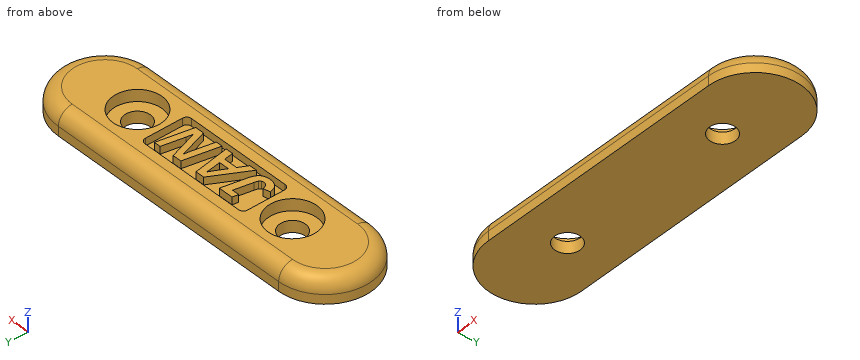
from build123d import *

# Parameters (mm, degrees)
F0_R     = 5.25
F0_R_2   = 2.75
F1_DEPTH = 5
F2_DEPTH = 2.5
F4_R     = 3
F6_DEPTH = 1.6


with BuildPart() as f1:
    # F0 (on Top) → F1 (new body)
    with BuildSketch(Plane.XY):
        with BuildLine():
            Line((27, 10), (-27, 10))
            ThreePointArc((-27, 10), (-37, 0), (-27, -10))
            Line((-27, -10), (27, -10))
            ThreePointArc((27, -10), (37, 0), (27, 10))
        make_face()
        with Locations((-19, 0)):
            Circle(F0_R, mode=Mode.SUBTRACT)
        with Locations((19, 0)):
            Circle(F0_R, mode=Mode.SUBTRACT)
        with Locations((-19, 0)):
            Circle(F0_R)
        with Locations((-19, 0)):
            Circle(F0_R_2, mode=Mode.SUBTRACT)
        with Locations((19, 0)):
            Circle(F0_R)
        with Locations((19, 0)):
            Circle(F0_R_2, mode=Mode.SUBTRACT)
    extrude(amount=-F1_DEPTH)

    # F0 (on Top) → F2 (cut)
    with BuildSketch(Plane.XY):
        with Locations((-19, 0)):
            Circle(F0_R)
        with Locations((-19, 0)):
            Circle(F0_R_2, mode=Mode.SUBTRACT)
        with Locations((19, 0)):
            Circle(F0_R)
        with Locations((19, 0)):
            Circle(F0_R_2, mode=Mode.SUBTRACT)
    extrude(amount=-F2_DEPTH, mode=Mode.SUBTRACT)

    # F4
    f4_edges = [f1.edges().sort_by_distance(p)[0] for p in [
        (0, -10, 0),
        (0, 10, 0),
    ]]
    fillet(f4_edges, radius=F4_R)

    # F5 (on face) → F6 (cut)
    with BuildSketch(Plane.XY):
        with BuildLine():
            Line((11.5, 5), (-11.5, 5))
            ThreePointArc((-11.5, 5), (-12.2071067812, 4.7071067812), (-12.5, 4))
            Line((-12.5, 4), (-12.5, -4))
            ThreePointArc((-12.5, -4), (-12.2071067812, -4.7071067812), (-11.5, -5))
            Line((-11.5, -5), (11.5, -5))
            ThreePointArc((11.5, -5), (12.2071067812, -4.7071067812), (12.5, -4))
            Line((12.5, -4), (12.5, 4))
            ThreePointArc((12.5, 4), (12.2071067812, 4.7071067812), (11.5, 5))
        make_face()
        with BuildLine():
            add(Edge.make_bspline(
                [(-7.1087151842, -3.5052785265), (-7.754492363, -4.0761455526), (-8.9168912848, -4.0761455526)],
                knots=[0, 0, 0, 1, 1, 1], degree=2))
            add(Edge.make_bspline(
                [(-8.9168912848, -4.0761455526), (-9.939802336, -4.0761455526), (-10.5502770291, -3.5586627733)],
                knots=[0, 0, 0, 1, 1, 1], degree=2))
            add(Edge.make_bspline(
                [(-10.5502770291, -3.5586627733), (-11.1607517221, -3.041179994), (-11.3656783468, -1.928721174)],
                knots=[0, 0, 0, 1, 1, 1], degree=2))
            Line((-11.3656783468, -1.928721174), (-9.9277478287, -1.6153039832))
            add(Edge.make_bspline(
                [(-9.9277478287, -1.6153039832), (-9.6814914645, -2.8328092243), (-8.8152890087, -2.8328092243)],
                knots=[0, 0, 0, 1, 1, 1], degree=2))
            add(Edge.make_bspline(
                [(-8.8152890087, -2.8328092243), (-8.5242587601, -2.8328092243), (-8.325359389, -2.7036537886)],
                knots=[0, 0, 0, 1, 1, 1], degree=2))
            add(Edge.make_bspline(
                [(-8.325359389, -2.7036537886), (-8.126460018, -2.5744983528), (-7.9973045822, -2.3377133872)],
                knots=[0, 0, 0, 1, 1, 1], degree=2))
            add(Edge.make_bspline(
                [(-7.9973045822, -2.3377133872), (-7.8681491465, -2.1009284217), (-7.7699910153, -1.5998053309)],
                knots=[0, 0, 0, 1, 1, 1], degree=2))
            Line((-7.7699910153, -1.5998053309), (-7.0002246181, 2.3712938005))
            Line((-7.0002246181, 2.3712938005), (-8.5139263252, 2.3712938005))
            Line((-8.5139263252, 2.3712938005), (-8.2762803235, 3.6146301288))
            Line((-8.2762803235, 3.6146301288), (-5.1817160827, 3.6146301288))
            Line((-5.1817160827, 3.6146301288), (-6.2201257862, -1.6910751722))
            add(Edge.make_bspline(
                [(-6.2201257862, -1.6910751722), (-6.4629380054, -2.9344115004), (-7.1087151842, -3.5052785265)],
                knots=[0, 0, 0, 1, 1, 1], degree=2))
        make_face(mode=Mode.SUBTRACT)
        Polygon((1.7909553759, -3.9676549865), (0.220425277, -3.9676549865), (-0.075771189, -2.0303234501), (-2.965408805, -2.0303234501), (-4.0141509434, -3.9676549865), (-5.5967355496, -3.9676549865), (-1.3621593291, 3.6146301288), (0.5114555256, 3.6146301288), align=None, mode=Mode.SUBTRACT)
        with BuildLine():
            Line((9.2613057802, -3.9676549865), (7.346361186, -3.9676549865))
            Line((7.346361186, -3.9676549865), (5.3332584606, 2.1181491465))
            add(Edge.make_bspline(
                [(5.3332584606, 2.1181491465), (5.2092692423, 1.2467804732), (5.1283318359, 0.8334830788)],
                knots=[0, 0, 0, 1, 1, 1], degree=2))
            Line((5.1283318359, 0.8334830788), (4.1915244085, -3.9676549865))
            Line((4.1915244085, -3.9676549865), (2.7828691225, -3.9676549865))
            Line((2.7828691225, -3.9676549865), (4.2569631626, 3.6146301288))
            Line((4.2569631626, 3.6146301288), (6.1409104522, 3.6146301288))
            Line((6.1409104522, 3.6146301288), (8.1695118299, -2.524558251))
            Line((8.1695118299, -2.524558251), (8.2332285115, -2.0837076969))
            add(Edge.make_bspline(
                [(8.2332285115, -2.0837076969), (8.2935010482, -1.6376909254), (8.3899371069, -1.1469002695)],
                knots=[0, 0, 0, 1, 1, 1], degree=2))
            Line((8.3899371069, -1.1469002695), (9.3267445343, 3.6146301288))
            Line((9.3267445343, 3.6146301288), (10.7353998203, 3.6146301288))
            Line((10.7353998203, 3.6146301288), (9.2613057802, -3.9676549865))
        make_face(mode=Mode.SUBTRACT)
        with BuildLine():
            add(Edge.make_bspline(
                [(-0.559673555, 1.596361186), (-0.6561096137, 2.3230757712), (-0.6561096137, 2.4470649895)],
                knots=[0, 0, 0, 1, 1, 1], degree=2))
            add(Edge.make_bspline(
                [(-0.6561096137, 2.4470649895), (-0.7697663971, 2.1026504942), (-1.184785864, 1.3070530099)],
                knots=[0, 0, 0, 1, 1, 1], degree=2))
            Line((-1.184785864, 1.3070530099), (-2.3247978437, -0.8352051512))
            Line((-2.3247978437, -0.8352051512), (-0.1997604073, -0.8352051512))
            Line((-0.1997604073, -0.8352051512), (-0.559673555, 1.596361186))
        make_face()
    extrude(amount=-F6_DEPTH, mode=Mode.SUBTRACT)


solid = f1.part
Source: CAD feature listing. Evaluate the final solid. Frame: model axes, mm. Give positions to 0.01 mm unless a question says otherwise; leave off trailing zeros. Write each loop counter-clockwise with the first axis right and the second up, starting at its lowest first coordinate (ties: lowest second). Pieces come first, ordered by that corner, then holes. Notation, with made-up numbers: M 9,18 L 44,18 A38 cw 44,56 Z; hole C 55.5,85 d6. An arc over 180 degrees is marked long. Return JSON: item names as keys, results as strings. Group by question number.
1) Cut plane B-B, the plane z = -4.1. Output: boundary loops of the cut face in (x, y).
2) Ray query, L1, parallel to X at y = 2.5, z = -3.6; L2, parallel to Y at x = 19, z = -4.25; L3, parallel to Y at x = -5, z = -0.45. Return the intervals inside material, ascending.
3) Cut plane C-C, the plane y = 0. Give the number of separate pieces and of enclosed holes in the cut face, then the cut area to 3 significant figures.
4) First-contact query: pin 1 Ø3 at (x, y) = (21.5, -2) entering from +Z; pin 2 Ø0.8 at (x, z) = (-8, -0.5) entering from -Y; pin 3 Ø1.3 at (x, z) = (-1.5, -1) entering from -Y; pin 4 Ø5 at (x, y) = (-19, 0) entering from -Z. Flat tips, straight axial feed; report the tip coordinate or a pass-through.
5) Cut plane A-A, the plane x = -19. Output: boundary loops of the cut face in (y, z).
Data:
{
 "1": {"outline": "M -27,-10 L 27,-10 A10 ccw 27,10 L -27,10 A10 ccw Z; hole C -19,0 d5.5; hole C 19,0 d5.5"},
 "2": {"L1": "x = -36.68 to -20.15, -17.85 to 17.85, 20.15 to 36.68", "L2": "y = -10 to -2.75, 2.75 to 10", "L3": "y = -8.58 to -5, -3.97 to -2.9, 5 to 8.58"},
 "3": {"separate pieces": "3", "enclosed holes": "0", "area": "260 mm²"},
 "4": {"pin 1": "stops at z = -2.5", "pin 2": "stops at y = -9.14", "pin 3": "stops at y = -9.68", "pin 4": "passes through"},
 "5": {"outline": "M -10,-5 L -2.75,-5 L -2.75,-2.5 L -5.25,-2.5 L -5.25,0 L -7,0 A3 ccw -10,-3 Z; M 2.75,-5 L 10,-5 L 10,-3 A3 ccw 7,0 L 5.25,0 L 5.25,-2.5 L 2.75,-2.5 Z"}
}
